from build123d import *

# Parameters (mm, degrees)
BOSS_EXTRUDE1_DEPTH = 40
SKETCH2_R           = 17.5
BOSS_EXTRUDE2_DEPTH = 34
CUT_EXTRUDE1_REACH  = 42
SKETCH3_R           = 3.167479455


with BuildPart() as part:
    # Sketch1 → Boss-Extrude1 (new body)
    with BuildSketch(Plane(origin=(0, 0, 0), x_dir=(1, 0, 0), z_dir=(0, 1, 0))):
        with BuildLine():
            Line((-29, 34), (29, 34))
            ThreePointArc((29, 34), (32.535533906, 32.535533906), (34, 29))
            Line((34, 29), (34, -29))
            ThreePointArc((34, -29), (32.535533906, -32.535533906), (29, -34))
            Line((29, -34), (-29, -34))
            ThreePointArc((-29, -34), (-32.535533906, -32.535533906), (-34, -29))
            Line((-34, -29), (-34, 29))
            ThreePointArc((-34, 29), (-32.535533906, 32.535533906), (-29, 34))
        make_face()
    extrude(amount=BOSS_EXTRUDE1_DEPTH)

    # Sketch2 → Boss-Extrude2 (add)
    with BuildSketch(Plane(origin=(0, 40, 0), x_dir=(1, 0, 0), z_dir=(0, 1, 0))):
        Circle(SKETCH2_R)
    extrude(amount=BOSS_EXTRUDE2_DEPTH)

    # Sketch3 → Cut-Extrude1 (cut, up to next)
    with BuildSketch(Plane(origin=(0, 40, 0), x_dir=(1, 0, 0), z_dir=(0, 1, 0)), mode=Mode.PRIVATE) as cut_extrude1_sk1:
        with Locations((-27.5, 27.5)):
            Circle(SKETCH3_R)
    cut_extrude1_tool1 = extrude(cut_extrude1_sk1.sketch, amount=-CUT_EXTRUDE1_REACH, mode=Mode.PRIVATE) & part.part
    add(cut_extrude1_tool1.solids().sort_by_distance((-27.5, 40, -27.5))[0], mode=Mode.SUBTRACT)
    # Sketch3 → Cut-Extrude1 (cut, up to next)
    with BuildSketch(Plane(origin=(0, 40, 0), x_dir=(1, 0, 0), z_dir=(0, 1, 0)), mode=Mode.PRIVATE) as cut_extrude1_sk2:
        with Locations((-27.5, -27.5)):
            Circle(SKETCH3_R)
    cut_extrude1_tool2 = extrude(cut_extrude1_sk2.sketch, amount=-CUT_EXTRUDE1_REACH, mode=Mode.PRIVATE) & part.part
    add(cut_extrude1_tool2.solids().sort_by_distance((-27.5, 40, 27.5))[0], mode=Mode.SUBTRACT)
    # Sketch3 → Cut-Extrude1 (cut, up to next)
    with BuildSketch(Plane(origin=(0, 40, 0), x_dir=(1, 0, 0), z_dir=(0, 1, 0)), mode=Mode.PRIVATE) as cut_extrude1_sk3:
        with Locations((27.5, -27.5)):
            Circle(SKETCH3_R)
    cut_extrude1_tool3 = extrude(cut_extrude1_sk3.sketch, amount=-CUT_EXTRUDE1_REACH, mode=Mode.PRIVATE) & part.part
    add(cut_extrude1_tool3.solids().sort_by_distance((27.5, 40, 27.5))[0], mode=Mode.SUBTRACT)
    # Sketch3 → Cut-Extrude1 (cut, up to next)
    with BuildSketch(Plane(origin=(0, 40, 0), x_dir=(1, 0, 0), z_dir=(0, 1, 0)), mode=Mode.PRIVATE) as cut_extrude1_sk4:
        with Locations((27.5, 27.5)):
            Circle(SKETCH3_R)
    cut_extrude1_tool4 = extrude(cut_extrude1_sk4.sketch, amount=-CUT_EXTRUDE1_REACH, mode=Mode.PRIVATE) & part.part
    add(cut_extrude1_tool4.solids().sort_by_distance((27.5, 40, -27.5))[0], mode=Mode.SUBTRACT)


solid = part.part
CAD build for the part. Positions are in the model's coordinates, mm. A direction names the side the tool comes from. Round coordinates to 2 decimals unless told otherwise and drop trailing zeros. Write each loop counter-clockwise with the first axis right and the second up, starting at its lowest first coordinate (ties: lowest second). Pieces come first, ordered by that corner, then holes. Notation, with made-up numbers: M 20,-1.75 L 66,-1.75 A27 ccw 66,30.25 Z; hole C -4.75,-7 d4. An arc over 180 degrees is marked long. Use a Markdown table: item, result. Add a question column.
1. Pull direction X, two halves, no side cores. Call faces 3 (the face through (-32, 20, 33)), 4 (the face through (-30.664, 20.28, 27.361)), 5 (the face through (0, 20, 34)), 6 (the face through (24.336, 20.28, -27.639)): released by +X, released by -X, zero draft, split by the parting line, or undercut.
2. Slice it at B-B on x = -27.5. Give the cut face in (y, z).
3. Drill centre lines: probe 1 along Z at (x, y) = (-27.5, 10); probe 2 along X at (y, z) = (23, -27). Where is each one in solid material? Low to high.
4. 3-axis set-ups, long thin cutter, end or side, ignore diameter. For faces 1 (the face through (24.99, 20.28, 29.43)), 2 (the face through (16, 40, -8)): which of +Z, -Z, +X, -X, +Y, -Y reach the whole face in a straight line?
5. Flat gauge pins, fed straight in: P1, Ø10, axis at x = 18, y = 55.5, coming from the -Z side; P2, Ø4, axis at x = -19, z = 12, coming from the +Y side; P3, Ø1.5, axis at x = 5, y = 49.5, coming from the -Z side. Where does each tip first touch, or does it go through?
6. Slice it at D-D on x = 0. Give the cut face in (y, z).
7. Slice it at C-C on y = 27. Give the cut face in (x, z).
8. Slice it at A-A on z = 27.5. Give the cut face in (x, y), then the cut area to 3 significant figures.
Reply:
| question | item | result |
|---|---|---|
| 1 | face 3 | released by -X |
| 1 | face 4 | undercut |
| 1 | face 5 | zero draft |
| 1 | face 6 | undercut |
| 2 | outline | M 0,-34 L 40,-34 L 40,-30.67 L 0,-30.67 Z; M 0,-24.33 L 40,-24.33 L 40,24.33 L 0,24.33 Z; M 0,30.67 L 40,30.67 L 40,34 L 0,34 Z |
| 3 | probe 1 | z = -34 to -30.67, -24.33 to 24.33, 30.67 to 34 |
| 3 | probe 2 | x = -34 to -30.63, -24.37 to 24.37, 30.63 to 34 |
| 4 | face 1 | +Y, -Y |
| 4 | face 2 | +Y |
| 5 | P1 | stops at z = -11.72 |
| 5 | P2 | stops at y = 40 |
| 5 | P3 | stops at z = -16.98 |
| 6 | outline | M 0,-34 L 40,-34 L 40,-17.5 L 74,-17.5 L 74,17.5 L 40,17.5 L 40,34 L 0,34 Z |
| 7 | outline | M -34,-29 A5 ccw -29,-34 L 29,-34 A5 ccw 34,-29 L 34,29 A5 ccw 29,34 L -29,34 A5 ccw -34,29 Z; hole C -27.5,-27.5 d6.33; hole C -27.5,27.5 d6.33; hole C 27.5,-27.5 d6.33; hole C 27.5,27.5 d6.33 |
| 8 | outline | M -34,0 L -30.67,0 L -30.67,40 L -34,40 Z; M -24.33,0 L 24.33,0 L 24.33,40 L -24.33,40 Z; M 30.67,0 L 34,0 L 34,40 L 30.67,40 Z |
| 8 | area | 2,210 mm^2 |
